Here's how the part is built. I have some questions about the finished solid (model axes, mm). Face numbers are marked on the shaded views. A direction names the side the tool comes from. Round coordinates to 2 decimals unless told otherwise and drop trailing zeros. Order: outer loops, then holes, each group sorted by start corner. A loop starts at its lowest first (then second) coordinate and runs counter-clockwise, first axis right, second up. Notation, with made-up numbers: (-40, 56) -> (-12, 56) arc R28 cw to (-12, 74) -> close; hole circle Ø2 at (-22, -7). An arc over 180 degrees is marked (long way). Answer in a Markdown table with one row per item.
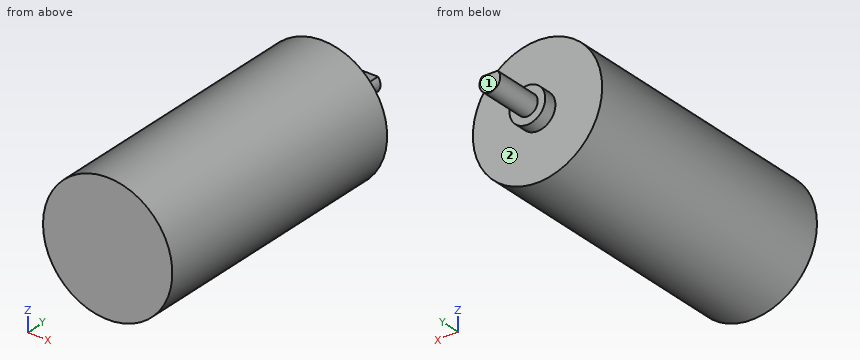
Autodesk Inventor part; units mm, degrees
ref_plane "YZ Plane" through (0, 0, 0) normal (1, 0, 0) x (0, 1, 0)
ref_plane "XZ Plane" through (0, 0, 0) normal (0, 1, 0) x (-1, 0, 0)
ref_plane "XY Plane" through (0, 0, 0) normal (0, 0, 1) x (1, 0, 0)
sketch "Sketch1" plane through (0, 0, 0) normal (0, 1, 0) x (-1, 0, 0)
  circle A0 centre (0, 0) radius 12.5
  dimension "d0" = 25
extrude "Extrusion1" add sketch "Sketch1" along normal blind 53.75
sketch "Sketch2" plane through (0, 53.75, 0) normal (0, 1, 0) x (1, 0, 0)
  circle A0 centre (0, 0) radius 2
  dimension "d3" = 4
extrude "Extrusion2" add sketch "Sketch2" along normal blind 11.938
sketch "Sketch3" plane through (0, 65.688, 0) normal (0, 1, 0) x (1, 0, 0)
  line L0 (-1.5129, -1.3081) -> (1.5129, -1.3081)
  circle A0 centre (0, 0) radius 2
  arc A1 (-1.5129, -1.3081) -> (1.5129, -1.3081) centre (0, 0) ccw
  dimension "d12" = 1.3081
extrude "Extrusion3" cut sketch "Sketch3" against normal up to surface (11.938 mm away) contours L0 A0 picked at (-0.3834, -1.4174)
sketch "Sketch4" plane through (0, 53.75, 0) normal (0, 1, 0) x (1, 0, 0)
  circle A0 centre (0, 0) radius 3.4607
  dimension "d9" = 6.9215
extrude "Extrusion4" add sketch "Sketch4" along normal blind 2.54
properties part number "Motor"
1. Suppose I cut it at B-B on z = 0. Write out the boundary of the cut face in (x, y), then the cut area to 3 significant figures.
Numbers:
| item | result |
|---|---|
| outline | (-12.5, 0) -> (12.5, 0) -> (12.5, 53.75) -> (3.46, 53.75) -> (3.46, 56.29) -> (2, 56.29) -> (2, 65.69) -> (-2, 65.69) -> (-2, 56.29) -> (-3.46, 56.29) -> (-3.46, 53.75) -> (-12.5, 53.75) -> close |
| area | 1,400 mm2 |
2. Please list where these lines run through material, in increasing order: line 1 along Y through (x, z) = (9, -6); line 2 along Y through (x, z) = (1.5, -2.25); line 3 along X through (y, z) = (32, 11.5).
Numbers:
| item | result |
|---|---|
| line 1 | y = 0 to 53.75 |
| line 2 | y = 0 to 56.29 |
| line 3 | x = -4.9 to 4.9 |
3. Suppose I cut it at C-C on y = 20.5. Write out the boundary of the cut face in (x, z), then the cut area to 3 significant figures.
Numbers:
| item | result |
|---|---|
| outline | circle Ø25 at (0, 0) |
| area | 491 mm2 |
4. For pin 1 Ø12 at (x, z) = (-7, 6) entering from +Y; pin 2 Ø4 at (x, z) = (6, -1.5) entering from +Y; pin 3 Ø5 at (x, z) = (3, 4) entering from -Y; pin 4 Ø10 at (x, y) = (-7, 40) entering from +Z, each with a flat end and sliding along its axis, tell me the tip position at first contact or that it passes through.
Numbers:
| item | result |
|---|---|
| pin 1 | stops at y = 56.29 |
| pin 2 | stops at y = 53.75 |
| pin 3 | stops at y = 0 |
| pin 4 | stops at z = 12.34 |
5. Suppose I cut it at D-D on y = 57.5. Write out the boundary of the cut face in (x, z), then the cut area to 3 significant figures.
Numbers:
| item | result |
|---|---|
| outline | (-1.51, 1.31) arc R2 ccw (long way) to (1.51, 1.31) -> close |
| area | 11.1 mm2 |
6. Suppose I cut it at A-A on x = 0. Write out the boundary of the cut face in (y, z).
Numbers:
| item | result |
|---|---|
| outline | (0, -12.5) -> (53.75, -12.5) -> (53.75, -3.46) -> (56.29, -3.46) -> (56.29, -2) -> (65.69, -2) -> (65.69, 1.31) -> (56.29, 1.31) -> (56.29, 3.46) -> (53.75, 3.46) -> (53.75, 12.5) -> (0, 12.5) -> close |
7. For the marked faces 1 and 2, which set-ups out of +Z, -Z, +X, -X, +Y, -Y let a thin tool reach every point of the face, with its end or its side?
Numbers:
| item | result |
|---|---|
| face 1 | +Z, -Z, +X, -X, +Y |
| face 2 | +Y |
